Check sheet for the drawn part. Datum: minimum x, y, z corner. Units: mm. Coordinates: 2 decimals unless noted, no trailing zeros. Order: outer loops, then holes, each group sorted by start corner. A loop starts at its lowest first (then second) coordinate and runs counter-clockwise, first axis right, second up.
1. Gauge pin test, flat ends, axial feed: pin 1 Ø1.9 at (x, y) = (2.59, 5.08) entering from +Z; pin 2 Ø3 at (x, y) = (7.03, 5.08) entering from +Z. Record the tip position at first contact, or that the pin passes through.
2. Cross-section at A-A (y = 5.08). Enter the section's corners in (x, z).
3. Cross-section at B-B (z = 2.45). Enter the section's corners in (x, y) (1 decimal).
4. Thickness scan on line 1 (X direction, y = 5.08, z = 1.5); line 2 (Y direction, x = 7, z = 2.95); line 3 (X direction, y = 4.5, z = 3.1). Record the ranges inside material, lowest first.
5. Draft check along X on the marked faces 1, 2, 3 and 4. Enter one of: released by +X, released by -X, zero draft, split by the parting line, or undercut.
6. Cross-section at D-D (x = 45.5). Enter the section's corners in (y, z) (1 decimal).
7. Cross-section at C-C (x = 7.5). Enter the section's corners in (y, z).
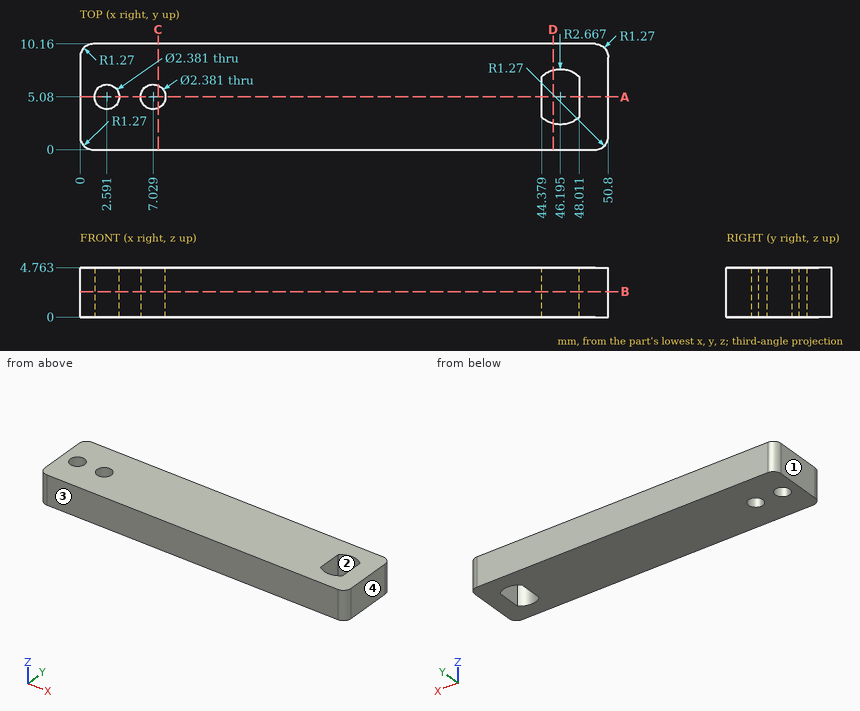
Data:
1. pin 1: passes through
1. pin 2: stops at z = 4.76
2. outline: (0, 0) - (1.4, 0) - (1.4, 4.76) - (0, 4.76) - close; (3.78, 0) - (5.84, 0) - (5.84, 4.76) - (3.78, 4.76) - close; (8.22, 0) - (44.38, 0) - (44.38, 4.76) - (8.22, 4.76) - close; (48.01, 0) - (50.8, 0) - (50.8, 4.76) - (48.01, 4.76) - close
3. outline: (0, 1.3) arc R1.3 ccw to (1.3, 0) - (49.5, 0) arc R1.3 ccw to (50.8, 1.3) - (50.8, 8.9) arc R1.3 ccw to (49.5, 10.2) - (1.3, 10.2) arc R1.3 ccw to (0, 8.9) - close; hole circle Ø2.4 at (2.6, 5.1); hole circle Ø2.4 at (7, 5.1); hole (44.4, 3.1) arc R2.7 ccw to (48, 3.1) - (48, 7) arc R2.7 ccw to (44.4, 7) - close
4. line 1: x = 0 to 1.4, 3.78 to 5.84, 8.22 to 44.38, 48.01 to 50.8
4. line 2: y = 0 to 3.89, 6.27 to 10.16
4. line 3: x = 0 to 1.55, 3.63 to 5.99, 8.07 to 44.38, 48.01 to 50.8
5. face 1: released by -X
5. face 2: undercut
5. face 3: zero draft
5. face 4: released by +X
6. outline: (0, 0) - (2.5, 0) - (2.5, 4.8) - (0, 4.8) - close; (7.7, 0) - (10.2, 0) - (10.2, 4.8) - (7.7, 4.8) - close
7. outline: (0, 0) - (3.99, 0) - (3.99, 4.76) - (0, 4.76) - close; (6.17, 0) - (10.16, 0) - (10.16, 4.76) - (6.17, 4.76) - close
